Geometry check sheet. Reference: the model listing, model coordinates, mm. Face numbers are marked on the shaded views. A direction names the side the tool comes from. Round coordinates to 2 decimals unless told otherwise and drop trailing zeros. Loops run counter-clockwise (first coordinate to the right, second up) from the corner with the lowest first, then second, coordinate; pieces in that order, holes last. Notation, with made-up numbers: M -20,-28.75 L 30,-28.75 A21 ccw 30,-20.75 Z; hole C -14,-29 d4. An arc over 180 degrees is marked long. Answer in a Markdown table with one row per item. Add a question column.
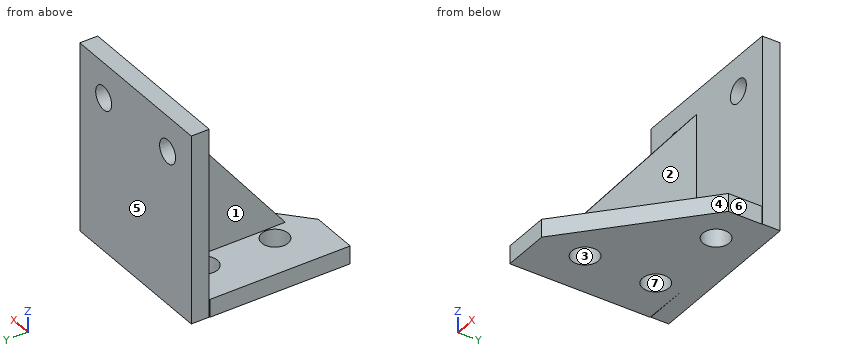
```python
from build123d import *

# Parameters (mm, degrees)
F0_R     = 7.112
F1_DEPTH = 9.652
F3_DEPTH = 2.47735
F4_W     = 88.9
F4_H     = 101.6
F4_R     = 6.35
F5_DEPTH = 9.652


with BuildPart() as f1:
    # F0 (on Top) → F1 (new body)
    with BuildSketch(Plane.XY):
        Polygon((54.822839, 34.332216), (-34.077161, 33.680932), (-34.077161, -41.867784), (-8.677161, -41.867784), (54.822839, 15.770677), align=None)
        with Locations((-10.201161, -17.488004)):
            Circle(F0_R, mode=Mode.SUBTRACT)
        with Locations((-10.201161, 20.611996)):
            Circle(F0_R, mode=Mode.SUBTRACT)
        with Locations((34.248839, 23.049973)):
            Circle(F0_R, mode=Mode.SUBTRACT)
    extrude(amount=F1_DEPTH)

    # F2 (on Right) → F3 (join, symmetric)
    with BuildSketch(Plane.YZ):
        Polygon((33.87592, 8.95272), (33.87592, 88.9), (-28.20982, 9.804583), align=None)
    extrude(amount=F3_DEPTH, both=True)

    # F4 (on face) → F5 (join)
    with BuildSketch(Plane(origin=(0, 33.87592, 0), x_dir=(-1, 0, 0), z_dir=(0, 1, 0))):
        with Locations((-10.612122, 50.8)):
            Rectangle(F4_W, F4_H)
        with Locations((-36.012122, 82.55)):
            Circle(F4_R, mode=Mode.SUBTRACT)
        with Locations((14.944623, 82.55)):
            Circle(F4_R, mode=Mode.SUBTRACT)
    extrude(amount=F5_DEPTH)


solid = f1.part
```
1) Set-up check for the marked faces 1, 2 and 3: record each of +Z, -Z, +X, -X, +Y, -Y from which the full face is reachable in a straight line by a thin tool's end or side.
2) Draft check along Y on the marked faces 4, 5, 6 and 7. Enter one of: +Y half, -Y half, draft (parallel to the pull), parting line (faces both ways), or undercut.
3) Thickness scan on L1, parallel to Z at x = 26, y = 33.5; L2, parallel to Y at x = 24, z = 72.5; L3, parallel to X at y = 35, z = 26.5. Record the ranges inside material, lowest first. Write a range as [from, to].
4) Cross-section at D-D, the plane x = 36. Record the boundary of the cut face in (y, z).
5) Cross-section at B-B, the plane z = 82.55. Record the boundary of the cut face in (x, y).
6) Cross-section at C-C, the plane x = -27. Record the boundary of the cut face in (y, z), plus the area to 3 significant figures.
7) Cross-section at A-A, the plane y = 26. Record the boundary of the cut face in (x, z).
8) Go/stop test with flat-tipped pins: pin 1 (14.5 mm diameter, centred on x = 36.01, z = 82.55, fed in from -Y); pin 2 (5 mm diameter, centred on y = 39.5, z = 65, fed in from -X); pin 3 (3 mm diameter, centred on y = 29.5, z = 4, fed in from +X); pin 4 (7.5 mm diameter, centred on x = -14.94, z = 82.55, fed in from +Y). Record where each tip stops, or that it passes through.
Worked answers:
| question | item | result |
|---|---|---|
| 1 | face 1 | +Z, -X, -Y |
| 1 | face 2 | +Z, +X, -Y |
| 1 | face 3 | +Z, -Z |
| 2 | face 4 | -Y half |
| 2 | face 5 | +Y half |
| 2 | face 6 | draft |
| 2 | face 7 | undercut |
| 3 | L1 | z = [0, 9.65] |
| 3 | L2 | y = [33.88, 43.53] |
| 3 | L3 | x = [-33.84, 55.06] |
| 4 | outline | M -1.31,0 L 16.16,0 L 16.16,9.65 L -1.31,9.65 Z; M 29.94,0 L 43.53,0 L 43.53,76.2 L 33.88,76.2 L 33.88,9.65 L 29.94,9.65 Z; M 33.88,88.9 L 43.53,88.9 L 43.53,101.6 L 33.88,101.6 Z |
| 5 | outline | M -33.84,33.88 L -21.29,33.88 L -21.29,43.53 L -33.84,43.53 Z; M -8.59,33.88 L -2.48,33.88 L -2.48,28.89 L 2.48,28.89 L 2.48,33.88 L 29.66,33.88 L 29.66,43.53 L -8.59,43.53 Z; M 42.36,33.88 L 55.06,33.88 L 55.06,43.53 L 42.36,43.53 Z |
| 6 | outline | M -41.87,0 L 33.73,0 L 33.73,9.65 L -41.87,9.65 Z; M 33.88,0 L 43.53,0 L 43.53,101.6 L 33.88,101.6 Z |
| 6 | area | 1,710 mm2 |
| 7 | outline | M -34.08,0 L -14.84,0 L -14.84,9.65 L -34.08,9.65 Z; M -5.56,0 L 27.78,0 L 27.78,9.65 L 2.48,9.65 L 2.48,78.87 L -2.48,78.87 L -2.48,9.65 L -5.56,9.65 Z; M 40.72,0 L 54.82,0 L 54.82,9.65 L 40.72,9.65 Z |
| 8 | pin 1 | stops at y = 33.88 |
| 8 | pin 2 | stops at x = -33.84 |
| 8 | pin 3 | stops at x = 54.82 |
| 8 | pin 4 | passes through |
